Source: CAD feature listing. Evaluate the final solid. Frame: model axes, mm. A direction names the side the tool comes from. Give positions to 0.01 mm unless a question says otherwise; leave off trailing zeros. Write each loop counter-clockwise with the first axis right and the second up, starting at its lowest first coordinate (ties: lowest second). Pieces come first, ordered by that corner, then holes. Notation, with made-up numbers: (18, -21) -> (57, -21) arc R26 ccw to (57, 7) -> close; hole circle Ø9 at (80, 36.5). An arc over 180 degrees is marked (long way). Answer as a JSON object with one key per item and string values. Group by question number.
Item 1: First-contact query: pin 1 Ø2.5 at (x, z) = (227, 19) entering from +Y; pin 2 Ø1.5 at (y, z) = (-25.5, 20.5) entering from -X; pin 3 Ø9 at (x, y) = (262.5, -13) entering from -Z. Flat tips, straight axial feed; report the tip coordinate or a pass-through.
Item 2: Section query A-A on x = 328. Return the cut outline in (y, z) (3 decimals).
Item 3: Section query C-C on y = -20.5. Return the cut outline in (x, z).
Item 4: Access query for faces 1 (the face through (250, -12, 24.899)), 2 (the face through (484.428, -29.932, 25.464)). Directions: +Z, -Z, +X, -X, +Y, -Y. A direction counts if a zero-diameter tool reaches every point of the face in a straight line with its end or side. Return the directions, or none.
Item 5: Section query B-B on z = 28.5. Return the cut outline in (x, y), plus the area to 3 significant figures.
Item 6: Ray query, probe 1 along Z at (x, y) = (146, -11.5); probe 2 along Y at (x, z) = (388, 24.75); probe 3 along X at (y, z) = (-20.5, 25.5). Return the intervals inside material, ascending. Write a range as from..to.
from build123d import *

# Parameters (mm, degrees)
F1_DEPTH = 558.8
F3_DEPTH = 19.178
F5_DEPTH = 19.178
F7_DEPTH = 19.178


with BuildPart() as f1:
    # F0 (on Right) → F1 (new body)
    with BuildSketch(Plane.YZ):
        with BuildLine():
            Line((-11.0857636662, 35.1864280597), (-48.1697636662, 35.1864280597))
            ThreePointArc((-48.1697636662, 35.1864280597), (-50.4148276965, 34.25649209), (-51.3447636662, 32.0114280597))
            Line((-51.3447636662, 32.0114280597), (-51.3447636662, 19.1844280597))
            ThreePointArc((-51.3447636662, 19.1844280597), (-50.4148276965, 16.9393640294), (-48.1697636662, 16.0094280597))
            Line((-48.1697636662, 16.0094280597), (-15.9117636662, 16.0094280597))
            Line((-15.9117636662, 16.0094280597), (-15.9117636662, 24.8994280597))
            Line((-15.9117636662, 24.8994280597), (-7.9107636662, 24.8994280597))
            Line((-7.9107636662, 24.8994280597), (-7.9107636662, 32.0114280597))
            ThreePointArc((-7.9107636662, 32.0114280597), (-8.8406996359, 34.25649209), (-11.0857636662, 35.1864280597))
        make_face()
    extrude(amount=F1_DEPTH)

    # F2 (on face) → F3 (cut, through all)
    with BuildSketch(Plane.XY.offset(35.1864280597)):
        Polygon((0, -11.0857636662), (40.259, -11.0857636662), (43.434, -7.9107636662), (0, -7.9107636662), align=None)
        Polygon((0, -48.1697636662), (3.175, -48.1697636662), (40.259, -11.0857636662), (0, -11.0857636662), align=None)
        Polygon((0, -48.1697636662), (0, -51.3447636662), (3.175, -48.1697636662), align=None)
    extrude(amount=-F3_DEPTH, mode=Mode.SUBTRACT)

    # F4 (on face) → F5 (cut, through all)
    with BuildSketch(Plane(origin=(0, 0, 16.0094280597), x_dir=(1, 0, 0), z_dir=(0, 0, -1))):
        Polygon((558.8, 48.1697636662), (558.8, 51.3447636662), (521.843, 51.3447636662), (518.668, 48.1697636662), align=None)
        Polygon((558.8, 15.9117636662), (558.8, 48.1697636662), (518.668, 48.1697636662), (486.41, 15.9117636662), align=None)
        Polygon((558.8, 7.9107636662), (558.8, 15.9117636662), (486.41, 15.9117636662), (478.409, 7.9107636662), align=None)
    extrude(amount=-F5_DEPTH, mode=Mode.SUBTRACT)

    # F6 (on face) → F7 (cut, through all)
    with BuildSketch(Plane(origin=(0, 0, 16.0094280597), x_dir=(1, 0, 0), z_dir=(0, 0, -1))):
        Polygon((470.408, 15.9117636662), (470.408, 15.5282095075), (470.408, 14.7099299356), (470.408, 7.9107636662), (478.409, 7.9107636662), (486.41, 15.9117636662), align=None)
        Polygon((470.408, 14.7099299356), (470.408, 15.5282095075), (470.408, 15.9117636662), (462.407, 7.9107636662), (470.408, 7.9107636662), align=None)
        Polygon((502.666, 48.1697636662), (470.408, 15.9117636662), (486.41, 15.9117636662), (518.668, 48.1697636662), align=None)
        Polygon((505.841, 51.3447636662), (502.666, 48.1697636662), (518.668, 48.1697636662), (521.843, 51.3447636662), align=None)
    extrude(amount=-F7_DEPTH, mode=Mode.SUBTRACT)


solid = f1.part
Worked answers:
{
 "1": {"pin 1": "y = -15.91", "pin 2": "x = 25.09", "pin 3": "z = 16.01"},
 "2": {"outline": "(-51.345, 19.184) arc R3.175 ccw to (-48.17, 16.009) -> (-15.912, 16.009) -> (-15.912, 24.899) -> (-7.911, 24.899) -> (-7.911, 32.011) arc R3.175 ccw to (-11.086, 35.186) -> (-48.17, 35.186) arc R3.175 ccw to (-51.345, 32.011) -> close"},
 "3": {"outline": "(30.84, 16.01) -> (475, 16.01) -> (475, 35.19) -> (30.84, 35.19) -> close"},
 "4": {"face 1": "-Z, +X, -X, +Y", "face 2": "+Z, -Z, +X, +Y"},
 "5": {"outline": "(0, -51.34) -> (505.84, -51.34) -> (462.41, -7.91) -> (43.43, -7.91) -> close", "area": "20,100 mm^2"},
 "6": {"probe 1": "24.9..35.19", "probe 2": "-51.34..-15.91", "probe 3": "30.84..475"}
}
